Verification items for the finished model (mm, model axes). Face numbers are marked on the shaded views. A direction names the side the tool comes from. Give positions to 0.01 mm unless a question says otherwise; leave off trailing zeros. Write each loop counter-clockwise with the first axis right and the second up, starting at its lowest first coordinate (ties: lowest second). Pieces come first, ordered by that corner, then holes. Notation, with made-up numbers: (-18.5, 2) -> (19.5, 2) arc R22 ccw to (19.5, 38) -> close; hole circle Ø3 at (-29.5, 64.5). An arc over 180 degrees is marked (long way). Answer as CSV lines item,"result".
```python
from build123d import *

# Parameters (mm, degrees)
BOSS_EXTRUDE1_DEPTH = 120
BOSS_EXTRUDE2_DEPTH = 15
CUT_EXTRUDE1_DEPTH  = 43
CUT_EXTRUDE2_DEPTH  = 43
FILLET1_R           = 3
FILLET2_R           = 3
SKETCH6_W           = 39.5
SKETCH6_H           = 23
SKETCH6_R           = 1.5
CUT_EXTRUDE3_DEPTH  = 3
SKETCH7_R           = 4.25
CUT_EXTRUDE4_DEPTH  = 2
SKETCH8_R           = 4.25
CUT_EXTRUDE5_DEPTH  = 2
BOSS_EXTRUDE3_START = 2
SKETCH9_R           = 4.25
BOSS_EXTRUDE3_DEPTH = 2
SKETCH10_R          = 2
BOSS_EXTRUDE4_DEPTH = 3


with BuildPart() as part:
    # Sketch2 → Boss-Extrude1 (new body)
    with BuildSketch(Plane.XY):
        Polygon((-18, 23), (0, 31.556461876), (18, 23), (18, 20), (18, 0), (21, 0), (21, 23), (0, 33), (-21, 23), (-21, 0), (-18, 0), (-18, 20), align=None)
    extrude(amount=BOSS_EXTRUDE1_DEPTH)

    # Sketch3 → Boss-Extrude2 (add)
    with BuildSketch(Plane.XY.offset(120)):
        Polygon((-18, 23), (-21, 23), (0, 33), (21, 23), (18, 23), (0, 31.556461876), align=None)
    extrude(amount=BOSS_EXTRUDE2_DEPTH)

    # Sketch4 → Cut-Extrude1 (cut)
    with BuildSketch(Plane.ZY.offset(21)):
        Polygon((135, 23), (120, 23), (135, 33), align=None)
    extrude(amount=-CUT_EXTRUDE1_DEPTH, mode=Mode.SUBTRACT)

    # Sketch5 → Cut-Extrude2 (cut)
    with BuildSketch(Plane(origin=(21, 0, 0), x_dir=(0, 0, -1), z_dir=(1, 0, 0))):
        Polygon((0, 23), (0, 33), (-10, 33), align=None)
    extrude(amount=-CUT_EXTRUDE2_DEPTH, mode=Mode.SUBTRACT)

    # Fillet1
    fillet1_edges = [part.edges().sort_by_distance(p)[0] for p in [
        (0, 33, 72.5),
    ]]
    fillet(fillet1_edges, radius=FILLET1_R)

    # Fillet2
    fillet2_edges = [part.edges().sort_by_distance(p)[0] for p in [
        (21, 23, 60),
    ]]
    fillet(fillet2_edges, radius=FILLET2_R)

    # Sketch6 → Cut-Extrude3 (cut)
    with BuildSketch(Plane.ZY.offset(21)):
        with Locations((26.75, 11.5)):
            Rectangle(SKETCH6_W, SKETCH6_H)
        with Locations((93.25, 11.5)):
            Rectangle(SKETCH6_W, SKETCH6_H)
        with Locations((116.5, 6.5)):
            Circle(SKETCH6_R)
        with Locations((116.5, 16.5)):
            Circle(SKETCH6_R)
        with Locations((70, 6.5)):
            Circle(SKETCH6_R)
        with Locations((50, 16.5)):
            Circle(SKETCH6_R)
        with Locations((3.5, 16.5)):
            Circle(SKETCH6_R)
        with Locations((3.5, 6.5)):
            Circle(SKETCH6_R)
        with Locations(Location((50, 6.5, 0), (0, 0, 180))):
            Circle(SKETCH6_R)
        with Locations((70, 16.5)):
            Circle(SKETCH6_R)
    extrude(amount=-CUT_EXTRUDE3_DEPTH, mode=Mode.SUBTRACT)

    # Sketch7 → Cut-Extrude4 (cut)
    with BuildSketch(Plane(origin=(21, 0, 0), x_dir=(0, 0, -1), z_dir=(1, 0, 0))):
        with Locations((-102.649161404, 10.552899521)):
            Circle(SKETCH7_R)
    extrude(amount=-CUT_EXTRUDE4_DEPTH, mode=Mode.SUBTRACT)

    # Sketch8 → Cut-Extrude5 (cut)
    with BuildSketch(Plane(origin=(21, 0, 0), x_dir=(0, 0, -1), z_dir=(1, 0, 0))):
        with Locations((-17.350838596, 10.552899521)):
            Circle(SKETCH8_R)
    extrude(amount=-CUT_EXTRUDE5_DEPTH, mode=Mode.SUBTRACT)

    # Sketch9 → Boss-Extrude3 (add)
    with BuildSketch(Plane(origin=(19, 0, 0), x_dir=(0, 0, -1), z_dir=(1, 0, 0)).offset(BOSS_EXTRUDE3_START)):
        with Locations((-17.350838596, 10.552899521)):
            Circle(SKETCH9_R)
    extrude(amount=-BOSS_EXTRUDE3_DEPTH)

    # Sketch10 → Boss-Extrude4 (add)
    with BuildSketch(Plane(origin=(21, 0, 0), x_dir=(0, 0, -1), z_dir=(1, 0, 0))):
        with Locations((-17.350838596, 10.552899521)):
            Circle(SKETCH10_R)
    extrude(amount=BOSS_EXTRUDE4_DEPTH)


solid = part.part
```
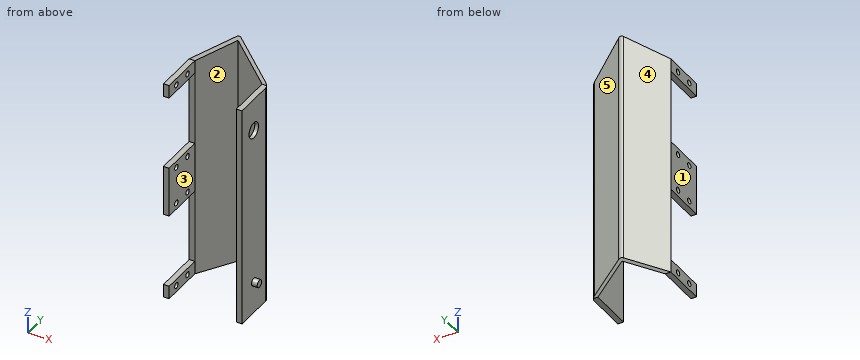
1) Draft check along X on the marked faces 3, 4 and 5. Enter one of: +X half, -X half, draft (parallel to the pull), parting line (faces both ways), or undercut.
Reported:
face 3,"undercut"
face 4,"-X half"
face 5,"+X half"
2) Tool access check on the marked faces 1 and 2. Record the directions out of +Z, -Z, +X, -X, +Y, -Y that give a thin tool (end or side, any length) a straight path to the whole face; none if there is none.
Reported:
face 1,"+Z, -Z, -X, +Y, -Y"
face 2,"+Z, -Z, -Y"
3) Scan lines: line 1 along Y through (x, z) = (-18.95, 3.5); line 2 along X through (y, z) = (3, 52); line 3 along Y through (x, z) = (-19.7, 50). Record each from-to range of solid material in increasing order.
Reported:
line 1,"0 to 5, 8 to 15, 18 to 23.98"
line 2,"-21 to -18, 18 to 21"
line 3,"0 to 5, 8 to 15, 18 to 23.62"
4) Section check C-C (z = 3.5). Record the boundary of the cut face in (x, y).
Reported:
outline,"(-21, 0) -> (-18, 0) -> (-18, 5) -> (-21, 5) -> close; (-21, 8) -> (-18, 8) -> (-18, 15) -> (-21, 15) -> close; (-21, 18) -> (-18, 18) -> (-18, 23) -> (-10.64, 26.5) -> (-13.65, 26.5) -> (-21, 23) -> close; (10.64, 26.5) -> (18, 23) -> (18, 0) -> (21, 0) -> (21, 21.11) arc R3 ccw to (19.29, 23.81) -> (13.65, 26.5) -> close"
5) Section check A-A (z = 70). Record the boundary of the cut face in (x, y).
Reported:
outline,"(-21, 0) -> (-18, 0) -> (-18, 5) -> (-21, 5) -> close; (-21, 8) -> (-18, 8) -> (-18, 15) -> (-21, 15) -> close; (-21, 18) -> (-18, 18) -> (-18, 23) -> (0, 31.56) -> (18, 23) -> (18, 0) -> (21, 0) -> (21, 21.11) arc R3 ccw to (19.29, 23.81) -> (1.29, 32.39) arc R3 ccw to (-1.29, 32.39) -> (-21, 23) -> close"
6) Section check B-B (y = 16.5). State how many separate pieces and enclosed holes the cut face has, and give its area (3 significant figures).
Reported:
separate pieces,"8"
enclosed holes,"0"
area,"447 mm²"
7) Section check D-D (z = 40). Record the boundary of the cut face in (x, y).
Reported:
outline,"(-21, 23) -> (-18, 23) -> (0, 31.56) -> (18, 23) -> (18, 0) -> (21, 0) -> (21, 21.11) arc R3 ccw to (19.29, 23.81) -> (1.29, 32.39) arc R3 ccw to (-1.29, 32.39) -> close"
8) Depth check by flat-ended pin: pin 1 (2.5 mm diameter, centred on y = 16.5, z = 50, fed in from -X); pin 2 (3.5 mm diameter, centred on x = -19.5, z = 36, fed in from -Y); pin 3 (5 mm diameter, centred on y = 16.5, z = 70, fed in from +X). Enter the tip coordinate at first touch or a pass-through.
Reported:
pin 1,"x = 18"
pin 2,"y = 23"
pin 3,"x = 21"
